Part model, mm, in its own coordinate system. A direction names the side the tool comes from. Round coordinates to 2 decimals unless told otherwise and drop trailing zeros. Order: outer loops, then holes, each group sorted by start corner. A loop starts at its lowest first (then second) coordinate and runs counter-clockwise, first axis right, second up. Notation, with made-up numbers: (88, 30) - (131, 30) arc R4 ccw to (131, 37) - close; hole circle Ø7 at (30.5, 65.25). An arc over 180 degrees is marked (long way). Return JSON: item names as keys, results as strings. Group by question number.
Item 1: Saw through at A-A on z = -3. State how many separate pieces and enclosed holes the cut face has, and give its area (3 significant figures).
Item 2: Saw through at B-B on y = 12.7. List the corners of the cut face in (x, z) (3 decimals).
Item 3: Tool access for faces 1 (the face through (-2.722, -18.573, 0.071)), 2 (the face through (-0.037, -5.897, 0.316)), 3 (the face through (-2.8, -6, 0.4)): list every direction of +Z, -Z, +X, -X, +Y, -Y with a clear straight run to the whole face (end or side of a thin tool).
Item 4: Probe probe 1 along Y at (x, z) = (0, 4); probe 2 along Y at (x, z) = (0, -2); probe 3 along Y at (x, z) = (-1.5, -4.75). List the from-to ranges inside material, lowest first.
Item 5: Drop flat-ended pins along their axis: pin 1 (1.2 mm diameter, centred on x = -0.5, y = 12.5, fed in from +Z); pin 2 (2.5 mm diameter, centred on y = 0, z = 3.175, fed in from +X). Give the stop position or say it passes through.
Item 6: Two-plate mould, pull along Z, no slides. Class faces 4 (the face through (2.21, 0.76, 2.34)), 5 (the face through (-0.31, -10.34, 4.06)), 6 (the face through (-2.503, -18.358, 5.355)): released by +Z, released by -Z, zero draft, split by the parting line, or undercut.
```python
from build123d import *

# Parameters (mm, degrees)
SKETCH1_W                                           = 6.35
SKETCH1_H                                           = 38.1
BOSS_EXTRUDE1_DEPTH                                 = 5.55625
SKETCH8_W                                           = 6.35
SKETCH8_H                                           = 12.7
CUT_EXTRUDE1_DEPTH                                  = 4.175
CUT_EXTRUDE1_DEPTH_BACK                             = 4.175
F_1_8_0_125_DIAMETER_HOLE1_D                        = 3.175
CBORE_FOR_2_BINDING_HEAD_MACHINE_SCREW2_D           = 2.4384
CBORE_FOR_2_BINDING_HEAD_MACHINE_SCREW2_CBORE_D     = 4.7625
CBORE_FOR_2_BINDING_HEAD_MACHINE_SCREW2_CBORE_DEPTH = 3.175
F_4_40_TAPPED_HOLE1_D                               = 2.2606
FILLET1_R                                           = 1.5875
FILLET2_R                                           = 0.396875
CHAMFER1_SIZE                                       = 0.508
CHAMFER2_SIZE                                       = 0.254


with BuildPart() as part:
    # Sketch1 → Boss-Extrude1 (new body, symmetric)
    with BuildSketch(Plane.XY):
        Rectangle(SKETCH1_W, SKETCH1_H)
    extrude(amount=BOSS_EXTRUDE1_DEPTH, both=True)

    # Sketch8 → Cut-Extrude1 (cut, two sides)
    with BuildSketch(Plane(origin=(0, 0, 0), x_dir=(0, 0, -1), z_dir=(1, 0, 0))) as cut_extrude1_sk:
        with Locations((2.38125, 0)):
            Rectangle(SKETCH8_W, SKETCH8_H)
    extrude(amount=CUT_EXTRUDE1_DEPTH, mode=Mode.SUBTRACT)
    extrude(cut_extrude1_sk.sketch, amount=-CUT_EXTRUDE1_DEPTH_BACK, mode=Mode.SUBTRACT)

    # 1/8 (0.125) Diameter Hole1 (through all)
    with Locations(Plane.XY.offset(5.55625)):
        with Locations((0, 0)):
            Hole(F_1_8_0_125_DIAMETER_HOLE1_D / 2)

    # CBORE for #2 Binding Head Machine Screw2 (through all)
    with Locations(Plane.XY.offset(5.55625)):
        with Locations((0, 12.7), (0, -12.7)):
            CounterBoreHole(CBORE_FOR_2_BINDING_HEAD_MACHINE_SCREW2_D / 2, CBORE_FOR_2_BINDING_HEAD_MACHINE_SCREW2_CBORE_D / 2, CBORE_FOR_2_BINDING_HEAD_MACHINE_SCREW2_CBORE_DEPTH)

    # #4-40 Tapped Hole1 (through all)
    with Locations(Plane(origin=(3.175, 0, 0), x_dir=(0, 0, -1), z_dir=(1, 0, 0))):
        with Locations((-3.175, 0)):
            Hole(F_4_40_TAPPED_HOLE1_D / 2)

    # Fillet1
    fillet1_edges = [part.edges().sort_by_distance(p)[0] for p in [
        (0, -6.35, 0.79375),
        (0, 6.35, 0.79375),
        (-3.175, -19.05, 0),
        (3.175, -19.05, 0),
        (3.175, 19.05, 0),
        (-3.175, 19.05, 0),
    ]]
    fillet(fillet1_edges, radius=FILLET1_R)

    # Fillet2
    fillet2_edges = [part.edges().sort_by_distance(p)[0] for p in [
        (-2.38125, -12.7, 2.38125),
        (-2.38125, 12.7, 2.38125),
    ]]
    fillet(fillet2_edges, radius=FILLET2_R)

    # Chamfer1
    chamfer1_edges = [part.edges().sort_by_distance(p)[0] for p in [
        (-3.175, 11.90625, -5.55625),
        (3.175, 11.90625, -5.55625),
        (0, 6.35, -5.55625),
        (0, -6.35, -5.55625),
        (-3.175, -6.35, -3.175),
        (3.175, -6.35, -3.175),
        (-3.175, 0, 0.79375),
        (3.175, 0, 0.79375),
        (-3.175, 6.35, -3.175),
        (3.175, 6.35, -3.175),
        (0, -19.05, -5.55625),
        (0, -19.05, 5.55625),
        (3.175, -11.90625, -5.55625),
        (-3.175, -11.90625, -5.55625),
        (2.710032015, -18.585032015, -5.55625),
        (-2.710032015, -18.585032015, -5.55625),
        (-3.175, 0, 5.55625),
        (3.175, 0, 5.55625),
        (0, 19.05, 5.55625),
        (2.710032015, 18.585032015, 5.55625),
        (-2.710032015, 18.585032015, 5.55625),
        (2.710032015, -18.585032015, 5.55625),
        (-2.710032015, -18.585032015, 5.55625),
        (0, 19.05, -5.55625),
        (2.710032015, 18.585032015, -5.55625),
        (-2.710032015, 18.585032015, -5.55625),
        (3.175, -5.885032015, 0.328782015),
        (-3.175, -5.885032015, 0.328782015),
        (3.175, 5.885032015, 0.328782015),
        (-3.175, 5.885032015, 0.328782015),
    ]]
    chamfer(chamfer1_edges, length=CHAMFER1_SIZE)

    # Chamfer2
    chamfer2_edges = [part.edges().sort_by_distance(p)[0] for p in [
        (1.5875, 0, 0.79375),
        (1.5875, 0, 5.55625),
        (-2.38125, -12.7, 5.55625),
        (1.2192, -12.7, -5.55625),
        (1.2192, -12.7, 2.38125),
        (-2.38125, 12.7, 5.55625),
        (1.2192, 12.7, -5.55625),
        (1.2192, 12.7, 2.38125),
        (-3.175, 0, 2.0447),
        (3.175, 0, 2.0447),
    ]]
    chamfer(chamfer2_edges, length=CHAMFER2_SIZE)


solid = part.part
```
Filled in:
{
 "1": {"separate pieces": "2", "enclosed holes": "2", "area": "149 mm^2"},
 "2": {"outline": "(-3.175, -5.048) - (-2.667, -5.556) - (-1.473, -5.556) - (-1.219, -5.302) - (-1.219, 2.127) - (-1.473, 2.381) - (-1.984, 2.381) arc R0.397 cw to (-2.381, 2.778) - (-2.381, 5.302) - (-2.635, 5.556) - (-2.667, 5.556) - (-3.175, 5.048) - close; (1.219, -5.302) - (1.473, -5.556) - (2.667, -5.556) - (3.175, -5.048) - (3.175, 5.048) - (2.667, 5.556) - (2.635, 5.556) - (2.381, 5.302) - (2.381, 2.778) arc R0.397 cw to (1.984, 2.381) - (1.473, 2.381) - (1.219, 2.127) - close"},
 "3": {"face 1": "+Z, -Z, -X, -Y", "face 2": "-Z, +X, -X", "face 3": "-Z, -X"},
 "4": {"probe 1": "y = -19.05 to -15.08, -10.32 to -1.59, 1.59 to 10.32, 15.08 to 19.05", "probe 2": "y = -19.05 to -13.92, -11.48 to -6.35, 6.35 to 11.48, 13.92 to 19.05", "probe 3": "y = -19.05 to -6.35, 6.35 to 19.05"},
 "5": {"pin 1": "passes through", "pin 2": "stops at x = 3.04"},
 "6": {"face 4": "undercut", "face 5": "zero draft", "face 6": "released by +Z"}
}
